CAD build for the part. Positions are in the model's coordinates, mm. Face numbers are marked on the shaded views. Coordinates: 2 decimals unless noted, no trailing zeros. Write each loop counter-clockwise with the first axis right and the second up, starting at its lowest first coordinate (ties: lowest second). Pieces come first, ordered by that corner, then holes. Notation, with made-up numbers: (34.25, 37) -> (88.25, 37) arc R15 cw to (88.25, 65) -> close; hole circle Ø7 at (-14, -12). An arc over 180 degrees is marked (long way). Answer as CSV lines item,"result".
```python
from build123d import *

# Parameters (mm, degrees)
SKETCH_1_W          = 135
SKETCH_1_H          = 100
EXTRUDE_1_DEPTH     = 20
SKETCH_2_R          = 1.7
CUT_EXTRUDE_1_DEPTH = 20
SKETCH_3_R          = 41.5
SKETCH_3_R_2        = 31
CUT_EXTRUDE_2_DEPTH = 6
SKETCH_4_R          = 2.5
CUT_EXTRUDE_3_DEPTH = 20


with BuildPart() as part:
    # 草图1 → 凸台-拉伸1 (new body)
    with BuildSketch(Plane.XY):
        Rectangle(SKETCH_1_W, SKETCH_1_H)
    extrude(amount=EXTRUDE_1_DEPTH)

    # 草图2 → 切除-拉伸1 (cut)
    with BuildSketch(Plane.XY.offset(20)):
        with Locations((14.159286998, 34.183542703)):
            Circle(SKETCH_2_R)
        with Locations((34.183542703, 14.159286998)):
            Circle(SKETCH_2_R)
        with Locations((34.183542703, -14.159286998)):
            Circle(SKETCH_2_R)
        with Locations((14.159286998, -34.183542703)):
            Circle(SKETCH_2_R)
        with Locations((-14.159286998, -34.183542703)):
            Circle(SKETCH_2_R)
        with Locations((-34.183542703, -14.159286998)):
            Circle(SKETCH_2_R)
        with Locations((-34.183542703, 14.159286998)):
            Circle(SKETCH_2_R)
        with Locations((-14.159286998, 34.183542703)):
            Circle(SKETCH_2_R)
    extrude(amount=-CUT_EXTRUDE_1_DEPTH, mode=Mode.SUBTRACT)

    # 草图3 → 切除-拉伸2 (cut)
    with BuildSketch(Plane.XY.offset(20)):
        Circle(SKETCH_3_R)
        Circle(SKETCH_3_R_2, mode=Mode.SUBTRACT)
    extrude(amount=-CUT_EXTRUDE_2_DEPTH, mode=Mode.SUBTRACT)

    # 草图4 → 切除-拉伸3 (cut)
    with BuildSketch(Plane.XY.offset(20)):
        with Locations((-60, 45)):
            Circle(SKETCH_4_R)
        with Locations((-50, 45)):
            Circle(SKETCH_4_R)
        with Locations((-55, 35)):
            Circle(SKETCH_4_R)
        with Locations((-40, 45)):
            Circle(SKETCH_4_R)
        with Locations((-45, 35)):
            Circle(SKETCH_4_R)
        with Locations((-30, 45)):
            Circle(SKETCH_4_R)
        with Locations((-35, 35)):
            Circle(SKETCH_4_R)
        with Locations((-50, 25)):
            Circle(SKETCH_4_R)
        with Locations((-55, 15)):
            Circle(SKETCH_4_R)
        with Locations((-60, 25)):
            Circle(SKETCH_4_R)
        with Locations((-45, 15)):
            Circle(SKETCH_4_R)
        with Locations(Location((45, 15, 0), (0, 0, 180))):
            Circle(SKETCH_4_R)
        with Locations(Location((60, 25, 0), (0, 0, 180))):
            Circle(SKETCH_4_R)
        with Locations(Location((55, 15, 0), (0, 0, 180))):
            Circle(SKETCH_4_R)
        with Locations(Location((50, 25, 0), (0, 0, 180))):
            Circle(SKETCH_4_R)
        with Locations(Location((35, 35, 0), (0, 0, 180))):
            Circle(SKETCH_4_R)
        with Locations(Location((30, 45, 0), (0, 0, 180))):
            Circle(SKETCH_4_R)
        with Locations(Location((45, 35, 0), (0, 0, 180))):
            Circle(SKETCH_4_R)
        with Locations(Location((40, 45, 0), (0, 0, 180))):
            Circle(SKETCH_4_R)
        with Locations(Location((55, 35, 0), (0, 0, 180))):
            Circle(SKETCH_4_R)
        with Locations(Location((50, 45, 0), (0, 0, 180))):
            Circle(SKETCH_4_R)
        with Locations(Location((60, 45, 0), (0, 0, 180))):
            Circle(SKETCH_4_R)
        with Locations((60, -45)):
            Circle(SKETCH_4_R)
        with Locations((50, -45)):
            Circle(SKETCH_4_R)
        with Locations((55, -35)):
            Circle(SKETCH_4_R)
        with Locations((40, -45)):
            Circle(SKETCH_4_R)
        with Locations((45, -35)):
            Circle(SKETCH_4_R)
        with Locations((30, -45)):
            Circle(SKETCH_4_R)
        with Locations((35, -35)):
            Circle(SKETCH_4_R)
        with Locations((50, -25)):
            Circle(SKETCH_4_R)
        with Locations((55, -15)):
            Circle(SKETCH_4_R)
        with Locations((60, -25)):
            Circle(SKETCH_4_R)
        with Locations((45, -15)):
            Circle(SKETCH_4_R)
        with Locations(Location((-45, -15, 0), (0, 0, 180))):
            Circle(SKETCH_4_R)
        with Locations(Location((-60, -25, 0), (0, 0, 180))):
            Circle(SKETCH_4_R)
        with Locations(Location((-55, -15, 0), (0, 0, 180))):
            Circle(SKETCH_4_R)
        with Locations(Location((-50, -25, 0), (0, 0, 180))):
            Circle(SKETCH_4_R)
        with Locations(Location((-35, -35, 0), (0, 0, 180))):
            Circle(SKETCH_4_R)
        with Locations(Location((-30, -45, 0), (0, 0, 180))):
            Circle(SKETCH_4_R)
        with Locations(Location((-45, -35, 0), (0, 0, 180))):
            Circle(SKETCH_4_R)
        with Locations(Location((-40, -45, 0), (0, 0, 180))):
            Circle(SKETCH_4_R)
        with Locations(Location((-55, -35, 0), (0, 0, 180))):
            Circle(SKETCH_4_R)
        with Locations(Location((-50, -45, 0), (0, 0, 180))):
            Circle(SKETCH_4_R)
        with Locations(Location((-60, -45, 0), (0, 0, 180))):
            Circle(SKETCH_4_R)
    extrude(amount=-CUT_EXTRUDE_3_DEPTH, mode=Mode.SUBTRACT)


solid = part.part
```
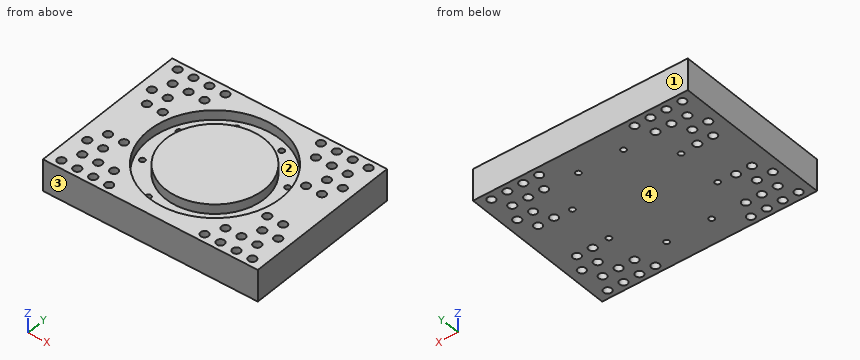
Item 1: Two-plate mould, pull along Y, no slides. Class the marked faces 1, 2, 3 and 4: pulls with the +Y half, pulls with the -Y half, needs draft (parallel to the pull), parting line crosses it, or undercut.
Answer below:
face 1,"pulls with the +Y half"
face 2,"undercut"
face 3,"pulls with the -Y half"
face 4,"needs draft"
Item 2: Saw through at D-D on x = 18. Give the cut face in (y, z), and give its area (3 significant figures).
Answer below:
outline,"(-50, 0) -> (50, 0) -> (50, 20) -> (37.39, 20) -> (37.39, 14) -> (25.24, 14) -> (25.24, 20) -> (-25.24, 20) -> (-25.24, 14) -> (-37.39, 14) -> (-37.39, 20) -> (-50, 20) -> close"
area,"1,850 mm2"
Item 3: Saw through at A-A on x = 60. Give the cut face in (y, z), and give its area (3 significant figures).
Answer below:
outline,"(-50, 0) -> (-47.5, 0) -> (-47.5, 20) -> (-50, 20) -> close; (-42.5, 0) -> (-27.5, 0) -> (-27.5, 20) -> (-42.5, 20) -> close; (-22.5, 0) -> (22.5, 0) -> (22.5, 20) -> (-22.5, 20) -> close; (27.5, 0) -> (42.5, 0) -> (42.5, 20) -> (27.5, 20) -> close; (47.5, 0) -> (50, 0) -> (50, 20) -> (47.5, 20) -> close"
area,"1,600 mm2"
Item 4: Saw through at C-C on y = 25. Give the cut face in (x, z), and give its area (3 significant figures).
Answer below:
outline,"(-67.5, 0) -> (-62.5, 0) -> (-62.5, 20) -> (-67.5, 20) -> close; (-57.5, 0) -> (-52.5, 0) -> (-52.5, 20) -> (-57.5, 20) -> close; (-47.5, 0) -> (47.5, 0) -> (47.5, 20) -> (33.12, 20) -> (33.12, 14) -> (18.33, 14) -> (18.33, 20) -> (-18.33, 20) -> (-18.33, 14) -> (-33.12, 14) -> (-33.12, 20) -> (-47.5, 20) -> close; (52.5, 0) -> (57.5, 0) -> (57.5, 20) -> (52.5, 20) -> close; (62.5, 0) -> (67.5, 0) -> (67.5, 20) -> (62.5, 20) -> close"
area,"2,120 mm2"
Item 5: Saw through at B-B on z = 16. State how many separate pieces and enclosed holes the cut face has, and give its area (3 significant figures).
Answer below:
separate pieces,"2"
enclosed holes,"45"
area,"10,200 mm2"
Item 6: Wall check: line 1 (Y direction, x = -50, z = 14.5); line 2 (Y direction, x = -30, z = 6.5); line 3 (Y direction, x = 45, z = 9.25). Give the ranges that are in metal, low to high. Write a range as from..to.
Answer below:
line 1,"y = -50..-47.5, -42.5..-27.5, -22.5..22.5, 27.5..42.5, 47.5..50"
line 2,"y = -50..-47.5, -42.5..42.5, 47.5..50"
line 3,"y = -50..-37.5, -32.5..-17.5, -12.5..12.5, 17.5..32.5, 37.5..50"
Item 7: Flat gauge pin, fed straight in: pin 1 (8 mm diameter, centred on x = -55, y = 35, fed in from +Z). Where does the tip first touch, or does it go through?
Answer below:
pin 1,"stops at z = 20"
